The figure shows three views and two pictorial views of one solid part (mm, origin at its lowest corner). Answer the questions. A direction names the side the tool comes from. Round coordinates to 2 decimals unless told otherwise and drop trailing zeros. Order: outer loops, then holes, each group sorted by start corner. A loop starts at its lowest first (then second) coordinate and runs counter-clockwise, first axis right, second up. Notation, with made-up numbers: M 5.25,20.25 L 26.25,20.25 A18 ccw 26.25,24.25 Z; hole C -40,18.25 d11. An arc over 180 degrees is marked long. Return JSON: item names as keys, results as strings.
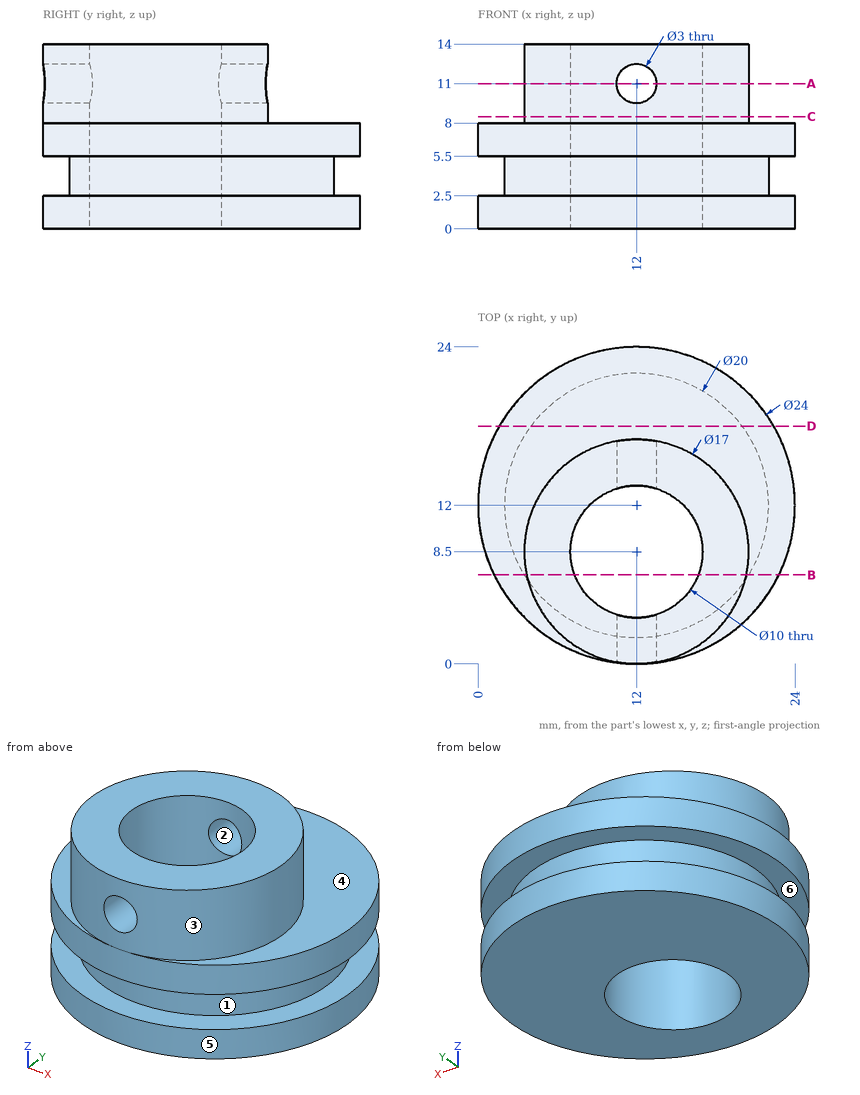
Item 1: Find section B-B (y = 6.75). Determine the outline of the cut face in (x, z).
Output:
{"outline": "M 1.21,0 L 7.32,0 L 7.32,14 L 3.68,14 L 3.68,8 L 1.21,8 L 1.21,5.5 L 3.49,5.5 L 3.49,2.5 L 1.21,2.5 Z; M 16.68,0 L 22.79,0 L 22.79,2.5 L 20.51,2.5 L 20.51,5.5 L 22.79,5.5 L 22.79,8 L 20.32,8 L 20.32,14 L 16.68,14 Z"}
Item 2: Find section A-A (z = 11). Determine the outline of the cut face in (x, y), plus the area to 3 significant figures.
Output:
{"outline": "M 10.5,0.13 L 10.5,3.73 A5 cw 10.5,13.27 L 10.5,16.87 A8.5 ccw Z; M 13.5,0.13 A8.5 ccw 13.5,16.87 L 13.5,13.27 A5 cw 13.5,3.73 Z", "area": "127 mm^2"}
Item 3: The mould has two halves that part along Z. Classify the marked faces 4, 5 and 6: pulls with the +Z half, pulls with the -Z half, needs draft (parallel to the pull), parting line crosses it, or undercut.
Output:
{"face 4": "pulls with the +Z half", "face 5": "needs draft", "face 6": "undercut"}
Item 4: Find section D-D (y = 18). Determine the outline of the cut face in (x, z), plus the area to 3 significant figures.
Output:
{"outline": "M 1.61,0 L 22.39,0 L 22.39,2.5 L 20,2.5 L 20,5.5 L 22.39,5.5 L 22.39,8 L 1.61,8 L 1.61,5.5 L 4,5.5 L 4,2.5 L 1.61,2.5 Z", "area": "152 mm^2"}
Item 5: Each of these flat-tipped pins is pushed along its axis until it touches: pin 1 (1.5 mm diameter, centred on y = 17, z = 10, fed in from -X); pin 2 (12 mm diameter, centred on x = 4, y = 21, fed in from +Z); pin 3 (3.5 mm diameter, centred on x = 12, z = 11, fed in from -Y); pin 4 (3 mm diameter, centred on x = 5, z = 3.5, fed in from +Y). Where does it stop, or does it pass through?
Output:
{"pin 1": "stops at x = 8.51", "pin 2": "stops at z = 8", "pin 3": "stops at y = 0", "pin 4": "stops at y = 22.46"}
Item 6: Which of the six approach directions +Z, -Z, +X, -X, +Y, -Y give full straight-line access (tool end or side, diameter ignored) to the marked faces 1, 2 and 3?
Output:
{"face 1": "none", "face 2": "+Y, -Y", "face 3": "+Z"}
Item 7: Find section C-C (z = 8.5). Determine the outline of the cut face in (x, y).
Output:
{"outline": "C 12,8.5 d17; hole C 12,8.5 d10"}
Item 8: Consider line 1 along Z through (x, y) = (12, 1.9); line 2 along Z through (x, y) = (7.5, 21.75); line 3 along Z through (x, y) = (3.25, 10.75). Determine where each line is inside the solid, lowest interval first. Write a range as [from, to].
Output:
{"line 1": "z = [0, 2.5], [5.5, 9.5], [12.5, 14]", "line 2": "z = [0, 2.5], [5.5, 8]", "line 3": "z = [0, 8]"}
